Geometry: see drawing. Coordinates: mm, zero at the bounding-box minimum. A direction names the side the tool comes from. Coordinates: 2 decimals unless noted, no trailing zeros. Order: outer loops, then holes, each group sorted by start corner. A loop starts at its lowest first (then second) coordinate and runs counter-clockwise, first axis right, second up. Notation, with made-up numbers: M -38.5,31 L -8.5,31 A26 ccw -8.5,48 Z; hole C 48,17.5 d1. An arc over 180 degrees is marked long. Answer in a Markdown table with one row per item.
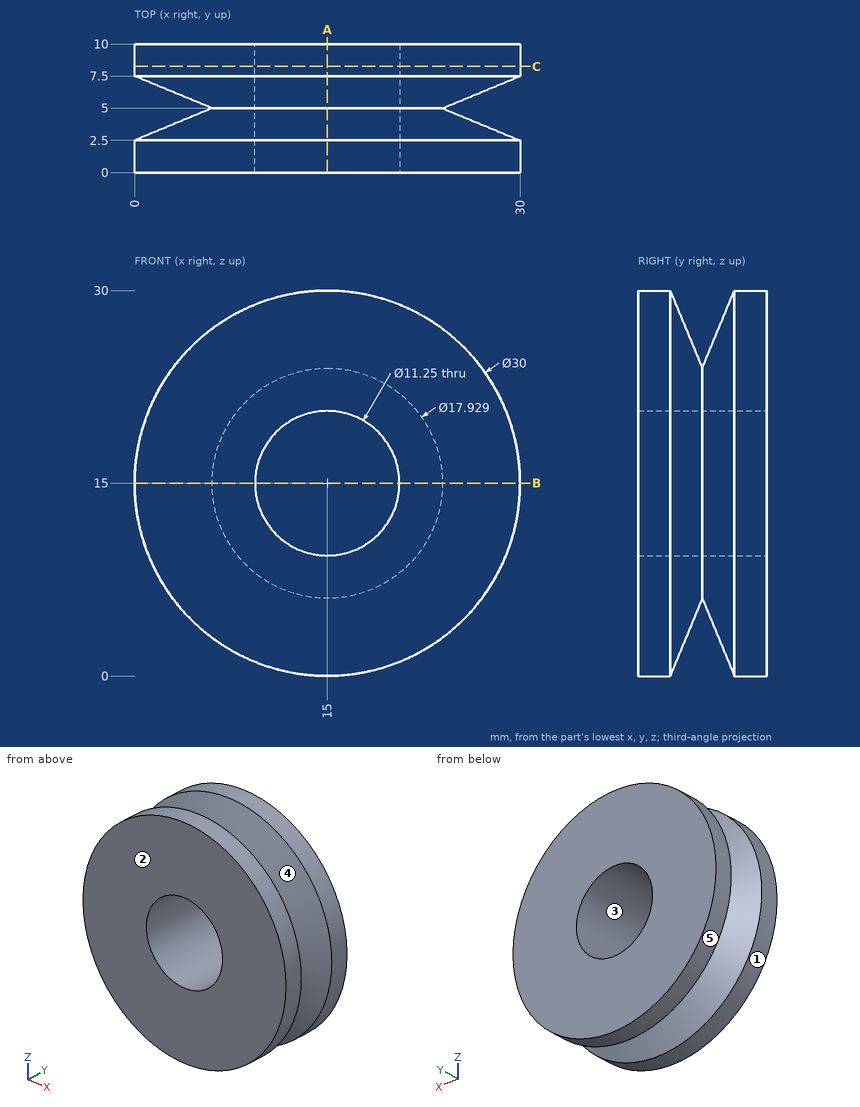
1) Reachability of the marked faces 4 and 5 from +Z, -Z, +X, -X, +Y, -Y: full face, straight path, thin tool, end or side. Return the list, or none.
Resolved:
| item | result |
|---|---|
| face 4 | none |
| face 5 | +Y, -Y |
2) Cut plane C-C, the plane y = 8.25. Output: boundary loops of the cut face in (x, z) (3 decimals), and give its area (3 significant figures).
Resolved:
| item | result |
|---|---|
| outline | C 15,15 d30; hole C 15,15 d11.25 |
| area | 607 mm2 |
3) Cut plane B-B, the plane z = 15. Output: boundary loops of the cut face in (x, y) (1 decimal), and give its area (3 significant figures).
Resolved:
| item | result |
|---|---|
| outline | M 0,0 L 9.4,0 L 9.4,10 L 0,10 L 0,7.5 L 6,5 L 0,2.5 Z; M 20.6,0 L 30,0 L 30,2.5 L 24,5 L 30,7.5 L 30,10 L 20.6,10 Z |
| area | 157 mm2 |
4) Material intervals for probe 1 along Z at (x, y) = (15, 9.5) (3 decimals); probe 2 along Z at (x, y) = (15, 4.5) (1 decimal); probe 3 along Y at (x, z) = (4, 17.5), sorted ascending.
Resolved:
| item | result |
|---|---|
| probe 1 | z = 0 to 9.375, 20.625 to 30 |
| probe 2 | z = 4.8 to 9.4, 20.6 to 25.2 |
| probe 3 | y = 0 to 4.04, 5.96 to 10 |
5) Mould query, pull axis Z, two halves, no side actions, for the marked faces 1, 2 and 3. Classes: +Z half, -Z half, draft (parallel to the pull), parting line (faces both ways), or undercut.
Resolved:
| item | result |
|---|---|
| face 1 | parting line |
| face 2 | draft |
| face 3 | undercut |
6) Cut plane A-A, the plane x = 15. Output: boundary loops of the cut face in (y, z) (1 decimal), and give its area (3 significant figures).
Resolved:
| item | result |
|---|---|
| outline | M 0,0 L 2.5,0 L 5,6 L 7.5,0 L 10,0 L 10,9.4 L 0,9.4 Z; M 0,20.6 L 10,20.6 L 10,30 L 7.5,30 L 5,24 L 2.5,30 L 0,30 Z |
| area | 157 mm2 |
7) Contact query for flat-ended pins moving along their axis: pin 1 (1 mm diameter, centred on y = 7.5, z = 23, fed in from -X); pin 2 (6 mm diameter, centred on x = 21, y = 1.5, fed in from +Z). Output: stop coordinate, or through.
Resolved:
| item | result |
|---|---|
| pin 1 | stops at x = 2.01 |
| pin 2 | stops at z = 29.7 |
